from build123d import *

# Parameters (mm, degrees)
BOSS_EXTRUDE1_DEPTH = 2
SKETCH2_W           = 17
SKETCH2_H           = 2
BOSS_EXTRUDE2_DEPTH = 5.5
SKETCH3_W           = 2.580637968
SKETCH3_H           = 2.580641016
SKETCH3_W_2         = 2.241280605
SKETCH3_H_2         = 2.241280605
SKETCH3_W_3         = 2.688165312
SKETCH3_H_3         = 2.580637968
SKETCH3_W_4         = 2.580640102
SKETCH3_H_4         = 2.68816836
SKETCH3_W_5         = 2.580641016
CUT_EXTRUDE1_DEPTH  = 5


with BuildPart() as part:
    # Sketch1 → Boss-Extrude1 (new body)
    with BuildSketch(Plane.XY):
        Polygon((-32.25, 0), (32.25, 0), (32.25, 3), (49.25, 3), (52.25, 6), (52.25, 23), (55.25, 23), (55.25, 32), (-55.25, 32), (-55.25, 23), (-52.25, 23), (-52.25, 6), (-49.25, 3), (-32.25, 3), align=None)
    extrude(amount=BOSS_EXTRUDE1_DEPTH)

    # Sketch2 → Boss-Extrude2 (add)
    with BuildSketch(Plane.XY.offset(2)):
        with Locations((-40.75, 4)):
            Rectangle(SKETCH2_W, SKETCH2_H)
        with Locations((40.75, 4)):
            Rectangle(SKETCH2_W, SKETCH2_H)
    extrude(amount=BOSS_EXTRUDE2_DEPTH)

    # Sketch3 → Cut-Extrude1 (cut)
    with BuildSketch(Plane(origin=(0, 0, 0), x_dir=(-1, 0, 0), z_dir=(0, 0, -1))):
        with Locations((3.81719709, 25.247293672)):
            Rectangle(SKETCH3_W, SKETCH3_H)
        with Locations((-22.915804717, 23.05138755)):
            Rectangle(SKETCH3_W_2, SKETCH3_H_2)
        Polygon((-21.451570254, 21.483859492), (-21.451570254, 17.935481524), (-21.490182318, 17.186866511), (-21.476760755, 16.797579304), (-21.386689002, 16.464291172), (-21.231630232, 16.327958094), (-20.947078705, 16.228780137), (-20.157604338, 16.139996469), (-19.354479198, 16.194152418), (-19.052864358, 16.273649135), (-18.873917192, 16.387460236), (-18.751023052, 16.692507734), (-18.724770323, 17.0838688), (-18.763403723, 17.82795418), (-18.763403723, 21.483859492), align=None)
        with Locations((16.980823721, 23.05138755)):
            Rectangle(SKETCH3_W_2, SKETCH3_H_2)
        Polygon((-13.60212352, 21.483859492), (-13.60212352, 13.419360508), (-21.451570254, 13.419360508), (-21.451570254, 5.46238582), (-18.763403723, 5.46238582), (-18.763403723, 10.838719492), (-13.60212352, 10.838719492), (-13.60212352, 5.46238582), (-8.225790152, 5.46238582), (-8.225790152, 8.043026836), (-11.021483418, 8.043026836), (-11.021483418, 21.483859492), align=None)
        Polygon((-8.010736988, 21.483859492), (-8.010736988, 16.215053164), (-5.430096887, 16.215053164), (-5.430096887, 18.903221524), (-2.741930356, 18.903221524), (-2.741930356, 8.15055418), (-0.161290254, 8.15055418), (-0.161290254, 18.903221524), (2.526878106, 18.903221524), (2.526878106, 21.483859492), align=None)
        with Locations((3.647518408, 17.335693467)):
            Rectangle(SKETCH3_W_2, SKETCH3_H_2)
        with Locations((9.13976709, 20.193540508)):
            Rectangle(SKETCH3_W_3, SKETCH3_H_3)
        Polygon((18.54834873, 21.483859492), (18.602112402, 17.936682436), (18.655876074, 14.387100508), (18.662800216, 13.409194818), (18.630388393, 12.40793962), (18.478863779, 11.42852517), (18.333504049, 10.96112961), (18.128450154, 10.516140508), (17.811648959, 10.023003064), (17.444951089, 9.593525234), (17.035386148, 9.227963049), (16.589983736, 8.926572846), (16.115772848, 8.689610963), (15.619783696, 8.517333736), (15.109044966, 8.409997806), (14.590586567, 8.367859206), (14.071437796, 8.391173968), (13.558628255, 8.480199038), (13.059187242, 8.635190142), (12.58014436, 8.856404229), (12.1285286, 9.144097024), (11.711370176, 9.498525474), (11.33569808, 9.919945307), (11.00854161, 10.408613164), (10.716068027, 11.052540045), (10.529929105, 11.749061994), (10.429370099, 12.483578178), (10.393636261, 13.241488372), (10.433622973, 14.76908745), (10.483849746, 16.215053164), (7.795684434, 16.215053164), (7.763966032, 14.373321414), (7.786948866, 12.471897633), (7.874330149, 11.531087627), (8.04183939, 10.614098351), (8.311627319, 9.733844181), (8.705844666, 8.903239492), (9.182301016, 8.190905738), (9.735606894, 7.557466415), (10.355845938, 7.004639682), (11.033102089, 6.534144306), (11.757459289, 6.14769814), (12.51900148, 5.84701995), (13.307812602, 5.633827895), (14.113976293, 5.509840132), (14.927576495, 5.476775123), (15.738697453, 5.536351331), (16.5374225, 5.690287218), (17.313836188, 5.940300638), (18.058021847, 6.288110356), (18.76006342, 6.735434531), (19.410045152, 7.283991321), (19.998050682, 7.935499492), (20.398488388, 8.506577954), (20.732234939, 9.110218504), (21.004927916, 9.742712337), (21.222204596, 10.400350341), (21.38970256, 11.07942371), (21.513059082, 11.776223637), (21.649898432, 13.208167331), (21.67782177, 14.666510058), (21.641929436, 16.121580758), (21.559096074, 18.903221524), (23.924682402, 18.903221524), (23.924682402, 21.483859492), align=None)
        with Locations((-25.752637039, 12.278477871)):
            Rectangle(SKETCH3_W_4, SKETCH3_H_4)
        Polygon((0.192376871, 7.784525328), (0.192274032, 5.543244726), (2.433554635, 5.543347565), (2.433657474, 7.784628168), align=None)
        with Locations((25.752636582, 6.752706328)):
            Rectangle(SKETCH3_W_5, SKETCH3_H)
    extrude(amount=-CUT_EXTRUDE1_DEPTH, mode=Mode.SUBTRACT)


solid = part.part
Could you check a few things on this model? Use its own coordinates, in mm. A direction names the side the tool comes from. Give positions to 0.01 mm unless a question says otherwise; leave off trailing zeros. Order: outer loops, then holes, each group sorted by start corner. A loop starts at its lowest first (then second) coordinate and runs counter-clockwise, first axis right, second up.
1. Suppose I cut it at D-D (x = 43). List the corners of the cut face in (y, z) for me, plus the area to 3 significant figures.
2. Suppose I cut it at A-A (z = 5.25). List the corners of the cut face in (x, y) for me, plus the area to 3 significant figures.
3. Will these pins go through, and if not, where does the flat tip stop? P1, Ø3, axis at x = 9.5, z = 5, coming from the -Y side; P2, Ø2, axis at y = 18, z = 0.5, coming from the +X side; P3, Ø1, axis at y = 20, z = 1, coming from the -X side; P4, Ø0.6, axis at y = 3.5, z = 5.5, coming from the -X side.
4. We'd pull the mould along X, two halves only. Please class faces 6 (the flat face through (-32.25, 2, 1)), 7 (the flat face through (54, 23, 1)), 8 (the flat face through (-15.86, 23, 1)): pulls with the +X half, pulls with the -X half, needs draft (parallel to the pull), parting line crosses it, or undercut.
5. For faces 1 (the flat face through (-23, 18.903, 1)), 2 (the flat face through (-32.25, 4, 5)), 3 (the flat face through (0, 0, 1)), 4 (the flat face through (41, 3, 4)), 5 (the flat face through (-41, 4, 7.5)), which set-ups out of +Z, -Z, +X, -X, +Y, -Y let a thin tool reach every point of the face, with its end or its side?
6. Suppose I cut it at B-B (y = 25.5). List the corners of the cut face in (x, z) for me.
7. I need wall thicknesses on L1, parallel to X at y = 13, z = 1.75; L2, parallel to X at y = 11, z = 1.25; L3, parallel to Y at x = 43, z = 4.75. Which ranges of each line are inside material? Lowest first, please.
8. Suppose I cut it at C-C (y = 20). List the corners of the cut face in (x, z) for me.
Solved:
1. outline: (3, 0) - (32, 0) - (32, 2) - (5, 2) - (5, 7.5) - (3, 7.5) - close
1. area: 69.0 mm2
2. outline: (-49.25, 3) - (-32.25, 3) - (-32.25, 5) - (-49.25, 5) - close; (32.25, 3) - (49.25, 3) - (49.25, 5) - (32.25, 5) - close
2. area: 68.0 mm2
3. P1: passes through
3. P2: stops at x = 52.25
3. P3: stops at x = -52.25
3. P4: stops at x = -49.25
4. face 6: pulls with the -X half
4. face 7: needs draft
4. face 8: undercut
5. face 1: +Z, -Z
5. face 2: +Z, +Y, -Y
5. face 3: +Z, -Z, +X, -X, -Y
5. face 4: +Z, -Z, +X, -Y
5. face 5: +Z, +X, -X, +Y, -Y
6. outline: (-55.25, 0) - (-5.11, 0) - (-5.11, 2) - (-55.25, 2) - close; (-2.53, 0) - (55.25, 0) - (55.25, 2) - (-2.53, 2) - close
7. L1: x = -52.25 to -21.63, -18.65 to -10.41, -7.78 to 0.16, 2.74 to 11.02, 21.45 to 24.46, 27.04 to 52.25
7. L2: x = -52.25 to -21.37, -18.35 to -10.74, -7.97 to 0.16, 2.74 to 11.02, 21.45 to 24.46, 27.04 to 52.25
7. L3: y = 3 to 5
8. outline: (-52.25, 0) - (-23.92, 0) - (-23.92, 2) - (-52.25, 2) - close; (-18.57, 0) - (-10.48, 0) - (-10.48, 2) - (-18.57, 2) - close; (-7.8, 0) - (-2.53, 0) - (-2.53, 2) - (-7.8, 2) - close; (8.01, 0) - (11.02, 0) - (11.02, 2) - (8.01, 2) - close; (13.6, 0) - (18.76, 0) - (18.76, 2) - (13.6, 2) - close; (21.45, 0) - (52.25, 0) - (52.25, 2) - (21.45, 2) - close
